from build123d import *

# Parameters (mm, degrees)
SKETCH2_R                  = 21
SKETCH2_W                  = 3.2
SKETCH2_H                  = 25.2
BOSS_EXTRUDE1_DEPTH        = 3
F_10_0_10_DIAMETER_HOLE1_D = 10
F_8_0_8_DIAMETER_HOLE1_D   = 8
F_12_0_12_DIAMETER_HOLE1_D = 12
CUT_EXTRUDE1_DEPTH         = 160.1679616
CUT_EXTRUDE1_DEPTH_BACK    = 160.1679616
SKETCH19_R                 = 0.5
CUT_EXTRUDE2_DEPTH         = 160.1679616
FILLET1_R                  = 0.5
F_6_0_6_DIAMETER_HOLE1_D   = 6


with BuildPart() as part:
    # Sketch2 → Boss-Extrude1 (new, symmetric)
    with BuildSketch(Plane.XY):
        Polygon((-68, 65), (95.2, 65), (110.2, 65), (110.2, -103), (0, -103), (-121.2, -103), (-121.2, 65), (-106.2, 65), align=None)
        Circle(SKETCH2_R, mode=Mode.SUBTRACT)
        with Locations((-77.6, 0)):
            Rectangle(SKETCH2_W, SKETCH2_H, mode=Mode.SUBTRACT)
        with Locations((66.6, 0)):
            Rectangle(SKETCH2_W, SKETCH2_H, mode=Mode.SUBTRACT)
    extrude(amount=BOSS_EXTRUDE1_DEPTH, both=True)

    # Ø10.0 (10) Diameter Hole1 (through all)
    with Locations(Plane.XY.offset(3)):
        with Locations((-68, 50), (-68, -55)):
            Hole(F_10_0_10_DIAMETER_HOLE1_D / 2)

    # Ø8.0 (8) Diameter Hole1 (through all)
    with Locations(Plane.XY.offset(3)):
        with Locations((-106.2, 50), (-106.2, -88), (95.2, -88), (95.2, 50)):
            Hole(F_8_0_8_DIAMETER_HOLE1_D / 2)

    # Ø12.0 (12) Diameter Hole1 (through all)
    with Locations(Plane.XY.offset(3)):
        with Locations((-45, 0), (45, 0)):
            Hole(F_12_0_12_DIAMETER_HOLE1_D / 2)

    # Sketch18 → Cut-Extrude1 (cut, two sides: drawn at the far end of the back side and taken through both)
    with BuildSketch(Plane(origin=(0, 0, -3), x_dir=(-1, 0, 0), z_dir=(0, 0, -1)).offset(-CUT_EXTRUDE1_DEPTH_BACK)):
        with BuildLine():
            Line((-60.867617043, -19.77708764), (-63.720786592, -20.704138623))
            ThreePointArc((-63.720786592, -20.704138623), (-3.506509068, -66.908178829), (61.207545662, -27.251355086))
            Line((61.207545662, -27.251355086), (58.466909289, -26.031145157))
            ThreePointArc((58.466909289, -26.031145157), (-3.3495012, -63.912290224), (-60.867617043, -19.77708764))
        make_face()
    extrude(amount=CUT_EXTRUDE1_DEPTH + CUT_EXTRUDE1_DEPTH_BACK, mode=Mode.SUBTRACT)

    # Sketch19 → Cut-Extrude2 (cut, through all)
    with BuildSketch(Plane(origin=(0, 0, -3), x_dir=(-1, 0, 0), z_dir=(0, 0, -1))):
        with Locations((-65, -12.6)):
            Circle(SKETCH19_R)
        with Locations((-68.2, -12.6)):
            Circle(SKETCH19_R)
        with Locations((-68.2, 12.6)):
            Circle(SKETCH19_R)
        with Locations((-65, 12.6)):
            Circle(SKETCH19_R)
        with Locations((79.2, -12.6)):
            Circle(SKETCH19_R)
        with Locations((76, -12.6)):
            Circle(SKETCH19_R)
        with Locations((79.2, 12.6)):
            Circle(SKETCH19_R)
        with Locations((76, 12.6)):
            Circle(SKETCH19_R)
    extrude(amount=-CUT_EXTRUDE2_DEPTH, mode=Mode.SUBTRACT)

    # Fillet1
    fillet1_edges = [part.edges().sort_by_distance(p)[0] for p in [
        (68.2, 12.1, 0),
        (68.2, -12.1, 0),
        (65.5, -12.6, 0),
        (65, 12.1, 0),
        (-76, -12.1, 0),
        (-76, 12.1, 0),
        (-78.7, -12.6, 0),
        (-79.2, 12.1, 0),
        (67.7, -12.6, 0),
        (67.7, 12.6, 0),
        (65.5, 12.6, 0),
        (-79.2, -12.1, 0),
        (-76.5, 12.6, 0),
        (-78.7, 12.6, 0),
        (-76.5, -12.6, 0),
        (65, -12.1, 0),
    ]]
    fillet(fillet1_edges, radius=FILLET1_R)

    # Ø6.0 (6) Diameter Hole1 (through all)
    with Locations(Plane.XY.offset(3)):
        with Locations((-49, -61), (52, -61)):
            Hole(F_6_0_6_DIAMETER_HOLE1_D / 2)


solid = part.part
Part model, mm, in its own coordinate system. A direction names the side the tool comes from. Give positions to 0.01 mm unless a question says otherwise; leave off trailing zeros. Loops run counter-clockwise (first coordinate to the right, second up) from the corner with the lowest first, then second, coordinate; pieces in that order, holes last. Notation, with made-up numbers: M 56.5,-22.5 L 76.5,-22.5 A25 cw 76.5,-0.5 Z; hole C -25.75,42.5 d11. An arc over 180 degrees is marked long. Put each result on its own line as item: value. Start each with the question number.
1) Saw through at B-B (x = 45). List the corners of the cut face in (y, z).
2) Saw through at C-C (z = -0.5). State how many separate pieces and enclosed holes the cut face has, then the cut area to 3 significant figures.
3) Probe probe 1 along X at (y, z) = (-87.5, 1.5); probe 2 along Y at (x, z) = (17.5, 1.25); probe 3 along Y at (x, z) = (45, -1.7). List the from-to ranges inside material, lowest first.
4) Pull direction X, two halves, no side cores. Call faces 3 (the flat face through (110.2, -18, 0)), 4 (the cylindrical face through (2.27, -63.96, 0.04)), 5 (the flat face through (-4, -36, -3)), 6 (the cylindrical face through (-67.349, -50.043, -0.042)): +X half, -X half, draft (parallel to the pull), parting line (faces both ways), or undercut.
5) Saw through at A-A (y = -44). List the corners of the cut face in (x, z), then the cut area to 3 significant figures.
6) 3-axis set-ups, long thin cutter, end or side, ignore diameter. For faces 1 (the cylindrical face through (4.63, -66.84, 0.04)), 2 (the flat face through (-4, 65, 0)): which of +Z, -Z, +X, -X, +Y, -Y reach the whole face in a straight line?
Numbers:
1. outline: M -103,-3 L -49.64,-3 L -49.64,3 L -103,3 Z; M -45.51,-3 L -6,-3 L -6,3 L -45.51,3 Z; M 6,-3 L 65,-3 L 65,3 L 6,3 Z
2. separate pieces: 1
2. enclosed holes: 14
2. area: 36,200 mm^2
3. probe 1: -121.2 to -110.17, -102.23 to 91.23, 99.17 to 110.2
3. probe 2: -103 to -64.67, -61.56 to -11.61, 11.61 to 65
3. probe 3: -103 to -49.64, -45.51 to -6, 6 to 65
4. face 3: +X half
4. face 4: undercut
4. face 5: draft
4. face 6: undercut
5. outline: M -121.2,-3 L -50.53,-3 L -50.53,3 L -121.2,3 Z; M -46.48,-3 L 46.48,-3 L 46.48,3 L -46.48,3 Z; M 50.53,-3 L 110.2,-3 L 110.2,3 L 50.53,3 Z
5. area: 1,340 mm^2
6. face 1: +Z, -Z
6. face 2: +Z, -Z, +X, -X, +Y
